from build123d import *

# Parameters (mm, degrees)
F1_DEPTH = 5
F2_R     = 5
F3_R     = 15


with BuildPart() as f1:
    # F0 (on Top) → F1 (new body)
    with BuildSketch(Plane.XY):
        Polygon((12.419975, -35.958487), (62.419975, -35.958487), (37.419975, 7.342783), align=None)
    extrude(amount=F1_DEPTH)

    # F2
    f2_edges = [f1.edges().sort_by_distance(p)[0] for p in [
        (62.419975, -35.958487, 2.5),
        (12.419975, -35.958487, 2.5),
    ]]
    fillet(f2_edges, radius=F2_R)

    # F3
    f3_edges = [f1.edges().sort_by_distance(p)[0] for p in [
        (37.419975, 7.342783, 2.5),
    ]]
    fillet(f3_edges, radius=F3_R)


solid = f1.part
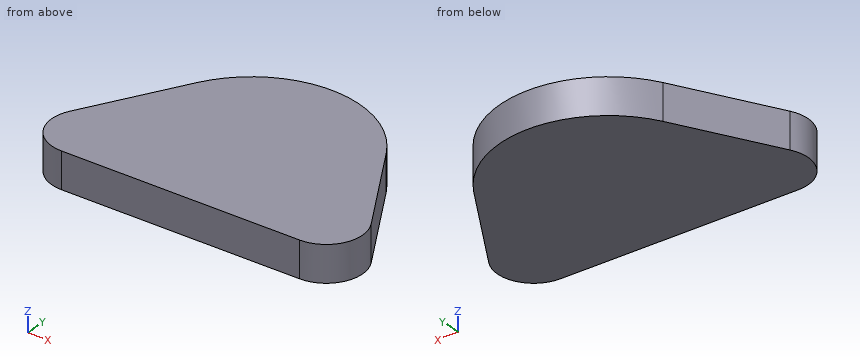
CAD build for the part. Positions are in the model's coordinates, mm. Round coordinates to 2 decimals unless told otherwise and drop trailing zeros. Order: outer loops, then holes, each group sorted by start corner. A loop starts at its lowest first (then second) coordinate and runs counter-clockwise, first axis right, second up. Notation, with made-up numbers: (34, -28) -> (65, -28) arc R21 ccw to (65, 8) -> close; hole circle Ø7 at (31, -38). An arc over 180 degrees is marked (long way). Write each question's results on one line, items separated by ' | '.
1. Cut at A-A (z = 0.45). Give the cut face in (x, y), plus the area to 3 significant figures.
Findings below:
outline: (16.75, -28.46) arc R5 ccw to (21.08, -35.96) -> (53.76, -35.96) arc R5 ccw to (58.09, -28.46) -> (50.41, -15.16) arc R15 ccw to (24.43, -15.16) -> close | area: 894 mm²
2. Cut at C-C (x = 48.5). Give the cut face in (y, z), plus the area to 3 significant figures.
Findings below:
outline: (-35.96, 0) -> (-12.55, 0) -> (-12.55, 5) -> (-35.96, 5) -> close | area: 117 mm²
3. Wall check: line 1 along X through (y, z) = (-13.5, 4.6); line 2 along X through (y, z) = (-12, 4.05); line 3 along Y through (x, z) = (36, 0.4). Give the ranges that are in metal, low to high. Write a range as [from, to].
Findings below:
line 1: x = [25.54, 49.3] | line 2: x = [26.86, 47.98] | line 3: y = [-35.96, -7.72]
4. Flat gauge pin, fed straight in: P1, Ø1, axis at y = -27, z = 2, coming from the -X side. Where does the tip first touch, or does it go through?
Findings below:
P1: stops at x = 17.3
5. Cut at B-B (y = -32.75). Give the cut face in (x, z), plus the area to 3 significant figures.
Findings below:
outline: (16.41, 0) -> (58.43, 0) -> (58.43, 5) -> (16.41, 5) -> close | area: 210 mm²
